Model file for the job. Use its own axes, mm. Face numbers are marked on the shaded views. A direction names the side the tool comes from. Round coordinates to 2 decimals unless told otherwise and drop trailing zeros. Order: outer loops, then holes, each group sorted by start corner. A loop starts at its lowest first (then second) coordinate and runs counter-clockwise, first axis right, second up. Notation, with made-up numbers: (80, 29) - (104, 29) arc R19 ccw to (104, 45) - close; hole circle Ø2 at (85, -8). An arc over 180 degrees is marked (long way). Put each result on its own line as item: value. Start each with the question number.
Item 1: Which spindle directions (+Z, -Z, +X, -X, +Y, -Y) get a long thin tool onto all of the face, cutting with end or side? Do the marked faces 4, 5 and 6. Say none if no direction does.
Item 2: Saw through at D-D on y = -8. List the corners of the cut face in (x, z).
Item 3: Saw through at A-A on y = 0. State how many separate pieces and enclosed holes the cut face has, plus the area to 3 significant figures.
Item 4: Pin check, flat tips, straight feed: pin 1 Ø2.5 at (y, z) = (0, 22.5) entering from -X; pin 2 Ø5 at (x, z) = (12.5, -3) entering from +Y. Stop position of each tip, or through.
Item 5: Mould opens along Y. For the marked faces 1, 2 and 3 say: pulls with the +Y half, pulls with the -Y half, needs draft (parallel to the pull), parting line crosses it, or undercut.
Item 6: Saw through at B-B on z = 7. List the corners of the cut face in (x, y), plus the area to 3 significant figures.
Item 7: Probe probe 1 along Y at (x, z) = (5, 11.5); probe 2 along Y at (x, z) = (14, 0). List the from-to ranges inside material, lowest first.
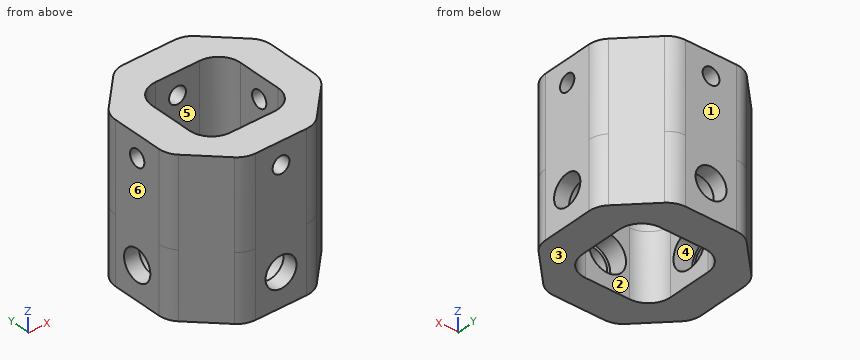
```python
from build123d import *

# Parameters (mm, degrees)
EXTRUDE_1_DEPTH          = 7.5
CUT_EXTRUDE_1_DEPTH      = 30.546573405
CUT_EXTRUDE_1_DEPTH_BACK = 30.546573405
SKETCH_2_W               = 20
SKETCH_2_H               = 20
SKETCH_11_W              = 29.504788154
SKETCH_11_H              = 47.493911142
CUT_EXTRUDE_7_DEPTH      = 0.4
SKETCH_12_W              = 20.237973212
SKETCH_12_H              = 25.719397838
CUT_EXTRUDE_8_DEPTH      = 0.4
FILLET_1_R               = 5
FILLET_2_R               = 5
CUT_EXTRUDE_2_DEPTH      = 41.063075269
CUT_EXTRUDE_2_DEPTH_BACK = 41.063075269
SKETCH_3_R               = 4.2
CUT_EXTRUDE_3_DEPTH      = 41.063075269
CUT_EXTRUDE_3_DEPTH_BACK = 41.063075269
SKETCH_4_R               = 4.2
EXTRUDE_2_DEPTH          = 20
SKETCH_6_R               = 4.2
SKETCH_6_R_2             = 3.5
EXTRUDE_3_DEPTH          = 3.4
EXTRUDE_START            = -3.4
SKETCH_13_R              = 4.2
SKETCH_13_R_2            = 3.5
EXTRUDE_4_DEPTH          = 3.4
SKETCH_14_R              = 1.9
CUT_EXTRUDE_9_DEPTH      = 49.010936254
SKETCH_15_R              = 1.9
CUT_EXTRUDE_10_DEPTH     = 49.010936254


with BuildPart() as part:
    # ｽｹｯﾁ1 → ﾎﾞｽ - 押し出し1 (new, symmetric)
    with BuildSketch(Plane.XY):
        Polygon((7.455844123, -18), (18, -7.455844123), (18, 7.455844123), (7.455844123, 18), (-7.455844123, 18), (-18, 7.455844123), (-18, -7.455844123), (-7.455844123, -18), align=None)
    extrude(amount=EXTRUDE_1_DEPTH, both=True)

    # ｽｹｯﾁ2 → ｶｯﾄ - 押し出し1 (cut, two sides: drawn at the far end of the back side and taken through both)
    with BuildSketch(Plane.XY.offset(7.5).offset(-CUT_EXTRUDE_1_DEPTH_BACK)):
        Rectangle(SKETCH_2_W, SKETCH_2_H)
    extrude(amount=CUT_EXTRUDE_1_DEPTH + CUT_EXTRUDE_1_DEPTH_BACK, mode=Mode.SUBTRACT)

    # ｽｹｯﾁ11 → ｶｯﾄ - 押し出し7 (cut)
    with BuildSketch(Plane(origin=(0, 18, 0), x_dir=(1, 0, 0), z_dir=(0, 1, 0))):
        Rectangle(SKETCH_11_W, SKETCH_11_H)
    cut_extrude_7 = extrude(amount=-CUT_EXTRUDE_7_DEPTH, mode=Mode.SUBTRACT)

    # ﾐﾗｰ1: ｶｯﾄ - 押し出し7 across plane
    add(cut_extrude_7.mirror(Plane.ZX), mode=Mode.SUBTRACT)

    # ｽｹｯﾁ12 → ｶｯﾄ - 押し出し8 (cut)
    with BuildSketch(Plane.ZY.offset(18)):
        Rectangle(SKETCH_12_W, SKETCH_12_H)
    cut_extrude_8 = extrude(amount=-CUT_EXTRUDE_8_DEPTH, mode=Mode.SUBTRACT)

    # ﾐﾗｰ2: ｶｯﾄ - 押し出し8 across plane
    add(cut_extrude_8.mirror(Plane(origin=(0, 0, 0), x_dir=(0, 0, 1), z_dir=(1, 0, 0))), mode=Mode.SUBTRACT)

    # ﾌｨﾚｯﾄ1
    fillet_1_edges = [part.edges().sort_by_distance(p)[0] for p in [
        (-10, -10, 0),
        (-10, 10, 0),
        (10, 10, 0),
        (10, -10, 0),
    ]]
    fillet(fillet_1_edges, radius=FILLET_1_R)

    # ﾌｨﾚｯﾄ2
    fillet_2_edges = [part.edges().sort_by_distance(p)[0] for p in [
        (17.6, 7.855844123, 0),
        (17.6, -7.855844123, 0),
        (-7.855844123, 17.6, 0),
        (7.855844123, 17.6, 0),
        (7.855844123, -17.6, 0),
        (-7.855844123, -17.6, 0),
        (-17.6, -7.855844123, 0),
        (-17.6, 7.855844123, 0),
    ]]
    fillet(fillet_2_edges, radius=FILLET_2_R)

    # ｽｹｯﾁ3 → ｶｯﾄ - 押し出し2 (cut, two sides: drawn at the far end of the back side and taken through both)
    with BuildSketch(Plane.XZ.offset(17.6).offset(-CUT_EXTRUDE_2_DEPTH_BACK)):
        with Locations(Location((0, 0, 0), (0, 0, 270))):
            Circle(SKETCH_3_R)
    extrude(amount=CUT_EXTRUDE_2_DEPTH + CUT_EXTRUDE_2_DEPTH_BACK, mode=Mode.SUBTRACT)

    # ｽｹｯﾁ4 → ｶｯﾄ - 押し出し3 (cut, two sides: drawn at the far end of the back side and taken through both)
    with BuildSketch(Plane(origin=(17.6, 0, 0), x_dir=(0, 0, -1), z_dir=(1, 0, 0)).offset(-CUT_EXTRUDE_3_DEPTH_BACK)):
        Circle(SKETCH_4_R)
    extrude(amount=CUT_EXTRUDE_3_DEPTH + CUT_EXTRUDE_3_DEPTH_BACK, mode=Mode.SUBTRACT)

    # ｽｹｯﾁ5 → ﾎﾞｽ - 押し出し2 (add)
    with BuildSketch(Plane.XY.offset(7.5)):
        with BuildLine():
            Line((17.6, -5.784776311), (17.6, 5.784776311))
            ThreePointArc((17.6, 5.784776311), (17.219397663, 7.698193473), (16.135533906, 9.320310217))
            Line((16.135533906, 9.320310217), (9.320310217, 16.135533906))
            ThreePointArc((9.320310217, 16.135533906), (7.698193473, 17.219397663), (5.784776311, 17.6))
            Line((5.784776311, 17.6), (-5.784776311, 17.6))
            ThreePointArc((-5.784776311, 17.6), (-7.698193473, 17.219397663), (-9.320310217, 16.135533906))
            Line((-9.320310217, 16.135533906), (-16.135533906, 9.320310217))
            ThreePointArc((-16.135533906, 9.320310217), (-17.219397663, 7.698193473), (-17.6, 5.784776311))
            Line((-17.6, 5.784776311), (-17.6, -5.784776311))
            ThreePointArc((-17.6, -5.784776311), (-17.219397663, -7.698193473), (-16.135533906, -9.320310217))
            Line((-16.135533906, -9.320310217), (-9.320310217, -16.135533906))
            ThreePointArc((-9.320310217, -16.135533906), (-7.698193473, -17.219397663), (-5.784776311, -17.6))
            Line((-5.784776311, -17.6), (5.784776311, -17.6))
            ThreePointArc((5.784776311, -17.6), (7.698193473, -17.219397663), (9.320310217, -16.135533906))
            Line((9.320310217, -16.135533906), (16.135533906, -9.320310217))
            ThreePointArc((16.135533906, -9.320310217), (17.219397663, -7.698193473), (17.6, -5.784776311))
        make_face()
        with BuildLine():
            Line((5, 10), (-5, 10))
            ThreePointArc((-5, 10), (-8.535533906, 8.535533906), (-10, 5))
            Line((-10, 5), (-10, -5))
            ThreePointArc((-10, -5), (-8.535533906, -8.535533906), (-5, -10))
            Line((-5, -10), (5, -10))
            ThreePointArc((5, -10), (8.535533906, -8.535533906), (10, -5))
            Line((10, -5), (10, 5))
            ThreePointArc((10, 5), (8.535533906, 8.535533906), (5, 10))
        make_face(mode=Mode.SUBTRACT)
    extrude(amount=EXTRUDE_2_DEPTH)

    # ｽｹｯﾁ6 → ﾎﾞｽ - 押し出し3 (add)
    with BuildSketch(Plane.XZ.offset(17.6)):
        Circle(SKETCH_6_R)
        Circle(SKETCH_6_R_2, mode=Mode.SUBTRACT)
    extrude_3 = extrude(amount=-EXTRUDE_3_DEPTH)

    # ﾐﾗｰ3: ﾎﾞｽ - 押し出し3 across plane
    add(extrude_3.mirror(Plane.ZX))

    # ｽｹｯﾁ13 → ﾎﾞｽ - 押し出し4 (add)
    with BuildSketch(Plane.ZY.offset(17.6).offset(EXTRUDE_START)):
        Circle(SKETCH_13_R)
        Circle(SKETCH_13_R_2, mode=Mode.SUBTRACT)
    extrude_4 = extrude(amount=EXTRUDE_4_DEPTH)

    # ﾐﾗｰ4: ﾎﾞｽ - 押し出し4 across plane
    add(extrude_4.mirror(Plane(origin=(0, 0, 0), x_dir=(0, 0, 1), z_dir=(1, 0, 0))))

    # ｽｹｯﾁ14 → ｶｯﾄ - 押し出し9 (cut, through all)
    with BuildSketch(Plane.ZY.offset(17.6)):
        with Locations((22.5, 0)):
            Circle(SKETCH_14_R)
    extrude(amount=-CUT_EXTRUDE_9_DEPTH, mode=Mode.SUBTRACT)

    # ｽｹｯﾁ15 → ｶｯﾄ - 押し出し10 (cut, through all)
    with BuildSketch(Plane.XZ.offset(17.6)):
        with Locations((0, 22.5)):
            Circle(SKETCH_15_R)
    extrude(amount=-CUT_EXTRUDE_10_DEPTH, mode=Mode.SUBTRACT)


solid = part.part
```
Results found:
1. face 4: none
1. face 5: +Z, -Z
1. face 6: +Z, -Z, -X, +Y, -Y
2. outline: (-17.08, -7.5) - (-9, -7.5) - (-9, 27.5) - (-17.08, 27.5) - close; (9, -7.5) - (17.08, -7.5) - (17.08, 27.5) - (9, 27.5) - close
3. separate pieces: 6
3. enclosed holes: 0
3. area: 356 mm²
4. pin 1: passes through
4. pin 2: stops at y = 15.46
5. face 1: pulls with the +Y half
5. face 2: undercut
5. face 3: needs draft
6. outline: (-17.6, -5.78) arc R5 ccw to (-16.14, -9.32) - (-9.32, -16.14) arc R5 ccw to (-5.78, -17.6) - (5.78, -17.6) arc R5 ccw to (9.32, -16.14) - (16.14, -9.32) arc R5 ccw to (17.6, -5.78) - (17.6, 5.78) arc R5 ccw to (16.14, 9.32) - (9.32, 16.14) arc R5 ccw to (5.78, 17.6) - (-5.78, 17.6) arc R5 ccw to (-9.32, 16.14) - (-16.14, 9.32) arc R5 ccw to (-17.6, 5.78) - close; hole (-10, -5) arc R5 ccw to (-5, -10) - (5, -10) arc R5 ccw to (10, -5) - (10, 5) arc R5 ccw to (5, 10) - (-5, 10) arc R5 ccw to (-10, 5) - close
6. area: 666 mm²
7. probe 1: y = -17.6 to -10, 10 to 17.6
7. probe 2: y = -11.46 to -4.2, 4.2 to 11.46
